```python
from build123d import *

# Parameters (mm, degrees)
F0_R     = 3.647768
F1_DEPTH = 570


with BuildPart() as f1:
    # F0 (on Front) → F1 (new body)
    with BuildSketch(Plane.XZ):
        with BuildLine():
            Line((-4.15, 22.5), (-22.5, 22.5))
            Line((-22.5, 22.5), (-22.5, 4.15))
            Line((-22.5, 4.15), (-18, 4.15))
            Line((-18, 4.15), (-18, 5.75))
            ThreePointArc((-18, 5.75), (-18.5, 6.25), (-18, 6.75))
            Line((-18, 6.75), (-9.8, 6.75))
            Line((-9.8, 6.75), (-7.2, 4.15))
            Line((-7.2, 4.15), (-7.2, -4.15))
            Line((-7.2, -4.15), (-9.8, -6.75))
            Line((-9.8, -6.75), (-18, -6.75))
            ThreePointArc((-18, -6.75), (-18.5, -6.25), (-18, -5.75))
            Line((-18, -5.75), (-18, -4.15))
            Line((-18, -4.15), (-22.5, -4.15))
            Line((-22.5, -4.15), (-22.5, -22.5))
            Line((-22.5, -22.5), (-4.15, -22.5))
            Line((-4.15, -22.5), (-4.15, -18))
            Line((-4.15, -18), (-5.75, -18))
            ThreePointArc((-5.75, -18), (-6.25, -18.5), (-6.75, -18))
            Line((-6.75, -18), (-6.75, -9.8))
            Line((-6.75, -9.8), (-4.15, -7.2))
            Line((-4.15, -7.2), (4.15, -7.2))
            Line((4.15, -7.2), (6.75, -9.8))
            Line((6.75, -9.8), (6.75, -18))
            ThreePointArc((6.75, -18), (6.25, -18.5), (5.75, -18))
            Line((5.75, -18), (4.15, -18))
            Line((4.15, -18), (4.15, -22.5))
            Line((4.15, -22.5), (22.5, -22.5))
            Line((22.5, -22.5), (22.5, -4.15))
            Line((22.5, -4.15), (18, -4.15))
            Line((18, -4.15), (18, -5.75))
            ThreePointArc((18, -5.75), (18.5, -6.25), (18, -6.75))
            Line((18, -6.75), (9.8, -6.75))
            Line((9.8, -6.75), (7.2, -4.15))
            Line((7.2, -4.15), (7.2, 4.15))
            Line((7.2, 4.15), (9.8, 6.75))
            Line((9.8, 6.75), (18, 6.75))
            ThreePointArc((18, 6.75), (18.5, 6.25), (18, 5.75))
            Line((18, 5.75), (18, 4.15))
            Line((18, 4.15), (22.5, 4.15))
            Line((22.5, 4.15), (22.5, 22.5))
            Line((22.5, 22.5), (4.15, 22.5))
            Line((4.15, 22.5), (4.15, 18))
            Line((4.15, 18), (5.75, 18))
            ThreePointArc((5.75, 18), (6.25, 18.5), (6.75, 18))
            Line((6.75, 18), (6.75, 9.8))
            Line((6.75, 9.8), (4.15, 7.2))
            Line((4.15, 7.2), (-4.15, 7.2))
            Line((-4.15, 7.2), (-6.75, 9.8))
            Line((-6.75, 9.8), (-6.75, 18))
            ThreePointArc((-6.75, 18), (-6.25, 18.5), (-5.75, 18))
            Line((-5.75, 18), (-4.15, 18))
            Line((-4.15, 18), (-4.15, 22.5))
        make_face()
        with BuildLine():
            Line((-8.9, -12.1), (-8.9, -19.5))
            ThreePointArc((-8.9, -19.5), (-9.192893, -20.207107), (-9.9, -20.5))
            Line((-9.9, -20.5), (-19.5, -20.5))
            ThreePointArc((-19.5, -20.5), (-20.207107, -20.207107), (-20.5, -19.5))
            Line((-20.5, -19.5), (-20.5, -9.9))
            ThreePointArc((-20.5, -9.9), (-20.207107, -9.192893), (-19.5, -8.9))
            Line((-19.5, -8.9), (-12.1, -8.9))
            Line((-12.1, -8.9), (-8.9, -12.1))
        make_face(mode=Mode.SUBTRACT)
        with BuildLine():
            Line((8.9, -12.1), (12.1, -8.9))
            Line((12.1, -8.9), (19.5, -8.9))
            ThreePointArc((19.5, -8.9), (20.207107, -9.192893), (20.5, -9.9))
            Line((20.5, -9.9), (20.5, -19.5))
            ThreePointArc((20.5, -19.5), (20.207107, -20.207107), (19.5, -20.5))
            Line((19.5, -20.5), (9.9, -20.5))
            ThreePointArc((9.9, -20.5), (9.192893, -20.207107), (8.9, -19.5))
            Line((8.9, -19.5), (8.9, -12.1))
        make_face(mode=Mode.SUBTRACT)
        with BuildLine():
            ThreePointArc((-20.5, 19.5), (-20.207107, 20.207107), (-19.5, 20.5))
            Line((-19.5, 20.5), (-9.9, 20.5))
            ThreePointArc((-9.9, 20.5), (-9.192893, 20.207107), (-8.9, 19.5))
            Line((-8.9, 19.5), (-8.9, 12.1))
            Line((-8.9, 12.1), (-12.1, 8.9))
            Line((-12.1, 8.9), (-19.5, 8.9))
            ThreePointArc((-19.5, 8.9), (-20.207107, 9.192893), (-20.5, 9.9))
            Line((-20.5, 9.9), (-20.5, 19.5))
        make_face(mode=Mode.SUBTRACT)
        Circle(F0_R, mode=Mode.SUBTRACT)
        with BuildLine():
            Line((12.1, 8.9), (8.9, 12.1))
            Line((8.9, 12.1), (8.9, 19.5))
            ThreePointArc((8.9, 19.5), (9.192893, 20.207107), (9.9, 20.5))
            Line((9.9, 20.5), (19.5, 20.5))
            ThreePointArc((19.5, 20.5), (20.207107, 20.207107), (20.5, 19.5))
            Line((20.5, 19.5), (20.5, 9.9))
            ThreePointArc((20.5, 9.9), (20.207107, 9.192893), (19.5, 8.9))
            Line((19.5, 8.9), (12.1, 8.9))
        make_face(mode=Mode.SUBTRACT)
    extrude(amount=F1_DEPTH)


solid = f1.part
```
Source: CAD feature listing. Evaluate the final solid. Frame: model axes, mm. A direction names the side the tool comes from. Round coordinates to 2 decimals unless told otherwise and drop trailing zeros.
(1) Access query for faces 4 (the flat face through (15, -281, -20.5)), 5 (the flat face through (-22.5, -281, -13)). Directions: +Z, -Z, +X, -X, +Y, -Y. A direction counts if a zero-diameter tool reaches every point of the face in a straight line with its end or side. Return the directions, or none.
From the geometry:
face 4: +Y, -Y
face 5: +Z, -Z, -X, +Y, -Y
(2) Material intervals for probe 1 along X at (y, z) = (-526, 14); probe 2 along X at (y, z) = (-248.5, 11), sorted ascending.
From the geometry:
probe 1: x = -22.5 to -20.5, -8.9 to -6.75, 6.75 to 8.9, 20.5 to 22.5
probe 2: x = -22.5 to -20.5, -10 to -6.75, 6.75 to 10, 20.5 to 22.5
(3) Contact query for a flat-ended pin moving along its axis: pin 1 Ø1 at (x, z) = (11.5, 5) entering from -Y. Output: stop coordinate, or through.
From the geometry:
pin 1: passes through
(4) Pull-direction query (Z, two-part tool) for faces 1 (the flat face through (-22.5, -281, 13)), 2 (the flat face through (13, -281, 22.5)), 3 (the flat face through (15, -281, 20.5)); classes: +Z half, -Z half, draft (parallel to the pull), parting line (faces both ways), or undercut.
From the geometry:
face 1: draft
face 2: +Z half
face 3: undercut
(5) Section query A-A (y = -244). Give the number of separate pieces and of enclosed holes in the cut face, and give its area (3 significant figures).
From the geometry:
separate pieces: 1
enclosed holes: 5
area: 759 mm2
